Input: part model. Units: mm. Frame: model coordinates. Coordinates: 2 decimals unless noted, no trailing zeros. Order: outer loops, then holes, each group sorted by start corner. A loop starts at its lowest first (then second) coordinate and runs counter-clockwise, first axis right, second up.
from build123d import *

# Parameters (mm, degrees)
SKETCH1_R           = 68.834
SKETCH1_R_2         = 65.659
BOSS_EXTRUDE1_DEPTH = 12.7
CUT_EXTRUDE1_START  = -68.834
SKETCH2_R           = 1.5875
CUT_EXTRUDE1_DEPTH  = 3.194194
CIRPATTERN1_COUNT   = 4
CHAMFER1_SIZE       = 1.27


with BuildPart() as part:
    # Sketch1 → Boss-Extrude1 (new body)
    with BuildSketch(Plane(origin=(0, 0, 0), x_dir=(1, 0, 0), z_dir=(0, 1, 0))):
        Circle(SKETCH1_R)
        Circle(SKETCH1_R_2, mode=Mode.SUBTRACT)
    extrude(amount=BOSS_EXTRUDE1_DEPTH)

    # Sketch2 → Cut-Extrude1 (cut)
    with BuildSketch(Plane.XY.offset(CUT_EXTRUDE1_START)):
        with Locations((0, 6.35)):
            Circle(SKETCH2_R)
    cut_extrude1 = extrude(amount=CUT_EXTRUDE1_DEPTH, mode=Mode.SUBTRACT)

    # CirPattern1: Cut-Extrude1 ×4 about axis
    cirpattern1_axis = Axis((0, 12.7, 0), (0, -1, 0))
    for i in range(1, CIRPATTERN1_COUNT):
        add(cut_extrude1.rotate(cirpattern1_axis, i * 360 / CIRPATTERN1_COUNT), mode=Mode.SUBTRACT)

    # Chamfer1
    chamfer1_edges = [part.edges().sort_by_distance(p)[0] for p in [
        (-65.659, 0, 0),
    ]]
    chamfer(chamfer1_edges, length=CHAMFER1_SIZE)


solid = part.part
Item 1: Pin query (flat end, axial travel): pin 1 Ø5 at (x, y) = (4.5, 9.5) entering from +Z. Return the tip coordinate at first contact, or that it passes through.
Response values:
pin 1: stops at z = 68.8
Item 2: Cut plane A-A on z = 0. Return loops of the section in (x, y).
Response values:
outline: (-68.83, 0) - (-66.93, 0) - (-65.66, 1.27) - (-65.66, 4.76) - (-68.83, 4.76) - close; (-68.83, 7.94) - (-65.66, 7.94) - (-65.66, 12.7) - (-68.83, 12.7) - close; (65.66, 1.27) - (66.93, 0) - (68.83, 0) - (68.83, 4.76) - (65.66, 4.76) - close; (65.66, 7.94) - (68.83, 7.94) - (68.83, 12.7) - (65.66, 12.7) - close
Item 3: Draft query along Z for faces 1 (the face through (61, 12.7, 25)), 2 (the face through (-14.9, 6.3, 67.2)), 3 (the face through (67.26, 4.94, 0.73)). Return one class per face: pulls with the +Z half, pulls with the -Z half, needs draft (parallel to the pull), parting line crosses it, or undercut.
Response values:
face 1: needs draft
face 2: parting line crosses it
face 3: undercut
Item 4: Cut plane B-B on x = 0. Return loops of the section in (y, z).
Response values:
outline: (0, -68.83) - (4.76, -68.83) - (4.76, -65.66) - (1.27, -65.66) - (0, -66.93) - close; (0, 66.93) - (1.27, 65.66) - (4.76, 65.66) - (4.76, 68.83) - (0, 68.83) - close; (7.94, -68.83) - (12.7, -68.83) - (12.7, -65.66) - (7.94, -65.66) - close; (7.94, 65.66) - (12.7, 65.66) - (12.7, 68.83) - (7.94, 68.83) - close
Item 5: Ray query, probe 1 along Y at (x, z) = (0, -67); probe 2 along X at (y, z) = (8.5, 0); probe 3 along Z at (x, y) = (43, 2). Return the intervals inside material, ascending.
Response values:
probe 1: y = 0 to 4.76, 7.94 to 12.7
probe 2: x = -68.83 to -65.66, 65.66 to 68.83
probe 3: z = -53.75 to -49.62, 49.62 to 53.75
Item 6: Cut plane C-C on y = 6.35. Return loops of the section in (x, z).
Response values:
outline: (-68.82, -1.59) arc R68.83 ccw to (-1.59, -68.82) - (-1.59, -65.64) arc R65.66 cw to (-65.64, -1.59) - close; (-68.82, 1.59) - (-65.64, 1.59) arc R65.66 cw to (-1.59, 65.64) - (-1.59, 68.82) arc R68.83 ccw to start; (1.59, -68.82) arc R68.83 ccw to (68.82, -1.59) - (65.64, -1.59) arc R65.66 cw to (1.59, -65.64) - close; (1.59, 65.64) arc R65.66 cw to (65.64, 1.59) - (68.82, 1.59) arc R68.83 ccw to (1.59, 68.82) - close
